from build123d import *

# Parameters (mm, degrees)
SKETCH1_R               = 3.5
BOSS_EXTRUDE1_DEPTH     = 6
FILLET1_R               = 2
SKETCH2_R               = 45
SKETCH2_R_2             = 40
BOSS_EXTRUDE2_DEPTH     = 6
FILLET2_R               = 2
SKETCH3_R               = 19
SKETCH3_R_2             = 14
BOSS_EXTRUDE3_DEPTH     = 6
FILLET3_R               = 2
SKETCH4_R               = 14
CUT_EXTRUDE1_DEPTH      = 2
SKETCH6_R               = 23
BOSS_EXTRUDE4_DEPTH     = 4
SKETCH7_R               = 7
CUT_EXTRUDE2_DEPTH      = 9
CUT_EXTRUDE2_DEPTH_BACK = 9


with BuildPart() as part:
    # Sketch1 → Boss-Extrude1 (new body)
    with BuildSketch(Plane(origin=(0, 0, 0), x_dir=(0, 0, -1), z_dir=(1, 0, 0))):
        with BuildLine():
            Line((59.755752861, 2.5), (32.04293994, 50.5))
            ThreePointArc((32.04293994, 50.5), (30.212812921, 52.330127019), (27.712812921, 53))
            Line((27.712812921, 53), (-27.712812921, 53))
            ThreePointArc((-27.712812921, 53), (-30.212812921, 52.330127019), (-32.04293994, 50.5))
            Line((-32.04293994, 50.5), (-59.755752861, 2.5))
            ThreePointArc((-59.755752861, 2.5), (-60.425625842, 0), (-59.755752861, -2.5))
            Line((-59.755752861, -2.5), (-32.04293994, -50.5))
            ThreePointArc((-32.04293994, -50.5), (-30.212812921, -52.330127019), (-27.712812921, -53))
            Line((-27.712812921, -53), (27.712812921, -53))
            ThreePointArc((27.712812921, -53), (30.212812921, -52.330127019), (32.04293994, -50.5))
            Line((32.04293994, -50.5), (59.755752861, -2.5))
            ThreePointArc((59.755752861, -2.5), (60.425625842, 0), (59.755752861, 2.5))
        make_face()
        with Locations((-51, 0)):
            Circle(SKETCH1_R, mode=Mode.SUBTRACT)
        with Locations((-25.5, 44.167295593)):
            Circle(SKETCH1_R, mode=Mode.SUBTRACT)
        with Locations((25.5, 44.167295593)):
            Circle(SKETCH1_R, mode=Mode.SUBTRACT)
        with Locations((51, 0)):
            Circle(SKETCH1_R, mode=Mode.SUBTRACT)
        with Locations((25.5, -44.167295593)):
            Circle(SKETCH1_R, mode=Mode.SUBTRACT)
        with Locations((-25.5, -44.167295593)):
            Circle(SKETCH1_R, mode=Mode.SUBTRACT)
    extrude(amount=BOSS_EXTRUDE1_DEPTH)

    # Fillet1
    fillet1_edges = [part.edges().sort_by_distance(p)[0] for p in [
        (0, 26.5, -45.899346401),
        (0, 0, -60.425625842),
        (0, -26.5, -45.899346401),
        (0, -52.330127019, -30.212812921),
        (0, -53, 0),
        (0, -52.330127019, 30.212812921),
        (0, -26.5, 45.899346401),
        (0, 0, 60.425625842),
        (0, 26.5, 45.899346401),
        (0, 52.330127019, 30.212812921),
        (0, 53, 0),
        (0, 52.330127019, -30.212812921),
    ]]
    fillet(fillet1_edges, radius=FILLET1_R)

    # Sketch2 → Boss-Extrude2 (add)
    with BuildSketch(Plane(origin=(6, 0, 0), x_dir=(0, 0, -1), z_dir=(1, 0, 0))):
        Circle(SKETCH2_R)
        Circle(SKETCH2_R_2, mode=Mode.SUBTRACT)
    extrude(amount=BOSS_EXTRUDE2_DEPTH)

    # Fillet2
    fillet2_edges = [part.edges().sort_by_distance(p)[0] for p in [
        (6, 0, 40),
    ]]
    fillet(fillet2_edges, radius=FILLET2_R)

    # Sketch3 → Boss-Extrude3 (add)
    with BuildSketch(Plane(origin=(6, 0, 0), x_dir=(0, 0, -1), z_dir=(1, 0, 0))):
        Circle(SKETCH3_R)
        Circle(SKETCH3_R_2, mode=Mode.SUBTRACT)
    extrude(amount=BOSS_EXTRUDE3_DEPTH)

    # Fillet3
    fillet3_edges = [part.edges().sort_by_distance(p)[0] for p in [
        (6, 0, 19),
    ]]
    fillet(fillet3_edges, radius=FILLET3_R)

    # Sketch4 → Cut-Extrude1 (cut)
    with BuildSketch(Plane(origin=(6, 0, 0), x_dir=(0, 0, -1), z_dir=(1, 0, 0))):
        Circle(SKETCH4_R)
    extrude(amount=-CUT_EXTRUDE1_DEPTH, mode=Mode.SUBTRACT)

    # Sketch6 → Boss-Extrude4 (add)
    with BuildSketch(Plane.ZY):
        Circle(SKETCH6_R)
    extrude(amount=BOSS_EXTRUDE4_DEPTH)

    # Sketch7 → Cut-Extrude2 (cut, two sides)
    with BuildSketch(Plane(origin=(4, 0, 0), x_dir=(0, 0, -1), z_dir=(1, 0, 0))) as cut_extrude2_sk:
        Circle(SKETCH7_R)
    extrude(amount=CUT_EXTRUDE2_DEPTH, mode=Mode.SUBTRACT)
    extrude(cut_extrude2_sk.sketch, amount=-CUT_EXTRUDE2_DEPTH_BACK, mode=Mode.SUBTRACT)


solid = part.part
CAD build for the part. Positions are in the model's coordinates, mm. A direction names the side the tool comes from. Round coordinates to 2 decimals unless told otherwise and drop trailing zeros. Loops run counter-clockwise (first coordinate to the right, second up) from the corner with the lowest first, then second, coordinate; pieces in that order, holes last. Notation, with made-up numbers: (34, 65) - (57, 65) arc R9 ccw to (57, 76) - close; hole circle Ø2 at (82, 28.25). An arc over 180 degrees is marked (long way). Put each result on its own line as item: value.
1. Wall check: line 1 (Y direction, x = 3.15, z = -25.5); line 2 (Y direction, x = 8.75, z = 0.5); line 3 (Z direction, x = 6.75, y = 12.5). Give the ranges that are in metal, low to high.
Geometry check:
line 1: -53 to -47.67, -40.67 to 40.67, 47.67 to 53
line 2: -45 to -40, -18.99 to -13.99, 13.99 to 18.99, 40 to 45
line 3: -43.23 to -37.53, -14.89 to -6.3, 6.3 to 14.89, 37.53 to 43.23
2. Two-plate mould, pull along Z, no slides. Class faces 1 (the cylindrical face through (9.97, -39.05, 8.67)), 2 (the cylindrical face through (3.972, -52.312, 30.244)), 3 (the cylindrical face through (0.6, -25.88, -45.6)): released by +Z, released by -Z, zero draft, split by the parting line, or undercut.
Geometry check:
face 1: undercut
face 2: released by +Z
face 3: released by -Z
3. 3-axis set-ups, long thin cutter, end or side, ignore diameter. For faces 4 (the cylindrical face through (9.972, -16.856, -8.767)), 5 (the cylindrical face through (-1.972, 22.804, -2.994)), 6 (the cylindrical face through (2.96, -47.27, 23.88)): which of +Z, -Z, +X, -X, +Y, -Y reach the whole face in a straight line?
Geometry check:
face 4: +X
face 5: -X
face 6: +X, -X
4. Slice it at B-B on x = -1.75. List the corners of the cut face in (y, z).
Geometry check:
outline: circle Ø46 at (0, 0); hole circle Ø14 at (0, 0)
5. Pin check, flat tips, straight feed: P1, Ø8, axis at y = 0, z = -51, coming from the -X side; P2, Ø12.5, axis at y = 0, z = 0, coming from the +X side; P3, Ø8, axis at x = 8, y = -32, coming from the +Z side; P4, Ø8, axis at x = -2, y = -5, coming from the +Z side. Stop position of each tip, or through.
Geometry check:
P1: x = 0
P2: through
P3: z = 44.72
P4: z = 59.53
6. Slice it at C-C on z = 25.5. Give the number of separate pieces and of enclosed holes in the cut face, and give its area (3 significant figures).
Geometry check:
separate pieces: 3
enclosed holes: 0
area: 628 mm²
